Here's how the part is built. I have some questions about the finished solid (model axes, mm). Give positions to 0.01 mm unless a question says otherwise; leave off trailing zeros. Write each loop counter-clockwise with the first axis right and the second up, starting at its lowest first coordinate (ties: lowest second). Pieces come first, ordered by that corner, then holes. Notation, with made-up numbers: (3.25, 74.5) -> (58.25, 74.5) arc R11 cw to (58.25, 78.5) -> close; hole circle Ø5 at (-21, 45.5). An arc over 180 degrees is marked (long way). Put each result on its own line as item: value. Start each with the question number.
from build123d import *

# Parameters (mm, degrees)
SKETCH1_W           = 2500
SKETCH1_H           = 284
BOSS_EXTRUDE1_DEPTH = 500
FILLET1_R           = 10
SKETCH2_W           = 2436
SKETCH2_H           = 220
CUT_EXTRUDE1_DEPTH  = 20
FILLET2_R           = 2


with BuildPart() as part:
    # Sketch1 → Boss-Extrude1 (new body)
    with BuildSketch(Plane.XY):
        with Locations((1250, 142)):
            Rectangle(SKETCH1_W, SKETCH1_H)
    extrude(amount=BOSS_EXTRUDE1_DEPTH)

    # Fillet1
    fillet1_edges = [part.edges().sort_by_distance(p)[0] for p in [
        (2500, 142, 500),
        (1250, 284, 500),
        (0, 142, 500),
        (1250, 284, 0),
        (2500, 142, 0),
        (1250, 0, 0),
        (0, 142, 0),
        (0, 284, 250),
        (2500, 284, 250),
        (2500, 0, 250),
        (0, 0, 250),
        (1250, 0, 500),
    ]]
    fillet(fillet1_edges, radius=FILLET1_R)

    # Sketch2 → Cut-Extrude1 (cut)
    with BuildSketch(Plane.XY.offset(500)):
        with Locations((1250, 142)):
            Rectangle(SKETCH2_W, SKETCH2_H)
    extrude(amount=-CUT_EXTRUDE1_DEPTH, mode=Mode.SUBTRACT)

    # Fillet2
    fillet2_edges = [part.edges().sort_by_distance(p)[0] for p in [
        (2468, 142, 480),
        (2468, 252, 490),
        (1250, 32, 480),
        (2468, 32, 490),
        (32, 142, 480),
        (32, 32, 490),
        (1250, 252, 480),
        (32, 252, 490),
        (2468, 142, 500),
        (1250, 252, 500),
        (32, 142, 500),
        (1250, 32, 500),
    ]]
    fillet(fillet2_edges, radius=FILLET2_R)


solid = part.part
1) Thinking about a two-plate mould opening in X: for faces 1 (the flat face through (1233, 144, 480)), 2 (the flat face through (1233, 0, 247)), 3 (the flat face through (0, 140, 247)), 4 (the flat face through (2500, 140, 247)), which applies, released by +X, released by -X, zero draft, split by the parting line, or undercut?
2) I need wall thicknesses on probe 1 along Z at (x, y) = (1792, 166). Which ranges of the line are inside material? Lowest first, please.
3) I want a section at A-A, the plane x = 1559. Write out the boundary of the cut face in (y, z).
4) I'm going to push a flat-ended pin straight in: pin 1 Ø3 at (x, y) = (273.5, 160.5) entering from +Z. Where does the tip first touch, or does it pass through?
5) I want a section at B-B, the plane y = 177.5. Write out the boundary of the cut face in (x, z), and give its area (3 significant figures).
Established:
1. face 1: undercut
1. face 2: zero draft
1. face 3: released by -X
1. face 4: released by +X
2. probe 1: z = 0 to 480
3. outline: (0, 10) arc R10 ccw to (10, 0) -> (274, 0) arc R10 ccw to (284, 10) -> (284, 490) arc R10 ccw to (274, 500) -> (254, 500) arc R2 ccw to (252, 498) -> (252, 482) arc R2 cw to (250, 480) -> (34, 480) arc R2 cw to (32, 482) -> (32, 498) arc R2 ccw to (30, 500) -> (10, 500) arc R10 ccw to (0, 490) -> close
4. pin 1: stops at z = 480
5. outline: (0, 10) arc R10 ccw to (10, 0) -> (2490, 0) arc R10 ccw to (2500, 10) -> (2500, 490) arc R10 ccw to (2490, 500) -> (2470, 500) arc R2 ccw to (2468, 498) -> (2468, 482) arc R2 cw to (2466, 480) -> (34, 480) arc R2 cw to (32, 482) -> (32, 498) arc R2 ccw to (30, 500) -> (10, 500) arc R10 ccw to (0, 490) -> close
5. area: 1,200,000 mm2
